Input: part model. Units: mm. Frame: model coordinates. Face numbers are marked on the shaded views. A direction names the side the tool comes from. Coordinates: 2 decimals unless noted, no trailing zeros. Loops run counter-clockwise (first coordinate to the right, second up) from the corner with the lowest first, then second, coordinate; pieces in that order, holes last. Notation, with made-up numbers: (45, 67.25) -> (89, 67.25) arc R14 ccw to (89, 74.25) -> close; hole circle Ø3 at (-22, 83.5). An arc over 180 degrees is marked (long way). Answer as a JSON object with one key per item and string values.
from build123d import *

# Parameters (mm, degrees)
F1_DEPTH = 15
F2_R     = 2


with BuildPart() as f1:
    # F0 (on Top) → F1 (new body)
    with BuildSketch(Plane.XY):
        Polygon((0, 30), (0, 0), (5, 0), (5, 15), (10.606602, 10.808817), (16.213203, 15), (16.213203, 0), (21.213203, 0), (21.213203, 30), (10.606602, 19.393398), align=None)
    extrude(amount=F1_DEPTH)

    # F2
    f2_edges = [f1.edges().sort_by_distance(p)[0] for p in [
        (15.909903, 24.696699, 15),
    ]]
    fillet(f2_edges, radius=F2_R)


solid = f1.part
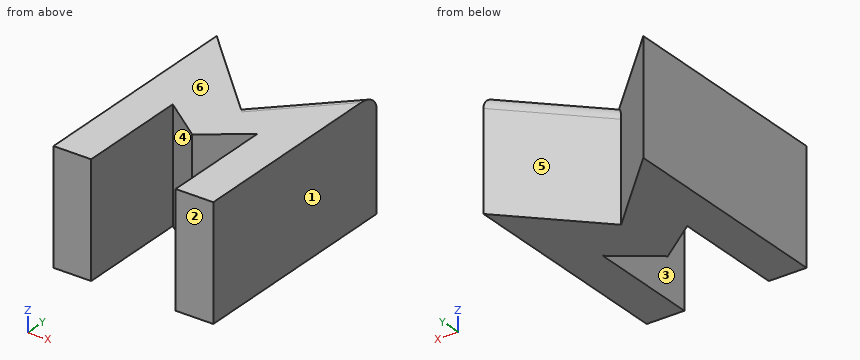
1. Pin query (flat end, axial travel): P1, Ø4, axis at x = 11.5, z = 2, coming from the +Y side; P2, Ø2, axis at x = 7.5, z = 3.5, coming from the -Y side; P3, Ø6, axis at x = 10, z = 10.5, coming from the +Y side. Return the tip coordinate at first contact, or that it passes through.
Reply:
{"P1": "stops at y = 22.29", "P2": "stops at y = 12.38", "P3": "stops at y = 23"}
2. Line query: line 1 along X through (y, z) = (3, 12.25); line 2 along X through (y, z) = (14.5, 11.5); line 3 along X through (y, z) = (26, 14). Output: solid intervals per line, ascending.
Reply:
{"line 1": "x = 0 to 5, 16.21 to 21.21", "line 2": "x = 0 to 5, 5.67 to 15.54, 16.21 to 21.21", "line 3": "x = 0 to 4, 17.59 to 21.21"}
3. Mould query, pull axis X, two halves, no side actions, for the marked faces 1, 2 and 3. Classes: pulls with the +X half, pulls with the -X half, needs draft (parallel to the pull), parting line crosses it, or undercut.
Reply:
{"face 1": "pulls with the +X half", "face 2": "needs draft", "face 3": "undercut"}
4. Section query D-D (x = 6.75). Return loops of the section in (y, z).
Reply:
{"outline": "(13.69, 0) -> (23.25, 0) -> (23.25, 15) -> (13.69, 15) -> close"}
5. Section query A-A (y = 2.5). Return loops of the section in (x, z), plus the area to 3 significant figures.
Reply:
{"outline": "(0, 0) -> (5, 0) -> (5, 15) -> (0, 15) -> close; (16.21, 0) -> (21.21, 0) -> (21.21, 15) -> (16.21, 15) -> close", "area": "150 mm2"}
6. Access query for the marked faces 4, 5 and 6. Directions: +Z, -Z, +X, -X, +Y, -Y. A direction counts if a zero-diameter tool reaches every point of the face in a straight line with its end or side. Return the directions, or none.
Reply:
{"face 4": "+Z, -Z, -Y", "face 5": "+Z, -Z, +Y", "face 6": "+Z, +X, -X, +Y, -Y"}
7. Section query B-B (z = 2.75). Return loops of the section in (x, y).
Reply:
{"outline": "(0, 0) -> (5, 0) -> (5, 15) -> (10.61, 10.81) -> (16.21, 15) -> (16.21, 0) -> (21.21, 0) -> (21.21, 30) -> (10.61, 19.39) -> (0, 30) -> close"}
8. Section query C-C (x = 9.25). Return loops of the section in (y, z), plus the area to 3 significant figures.
Reply:
{"outline": "(11.82, 0) -> (20.75, 0) -> (20.75, 15) -> (11.82, 15) -> close", "area": "134 mm2"}
